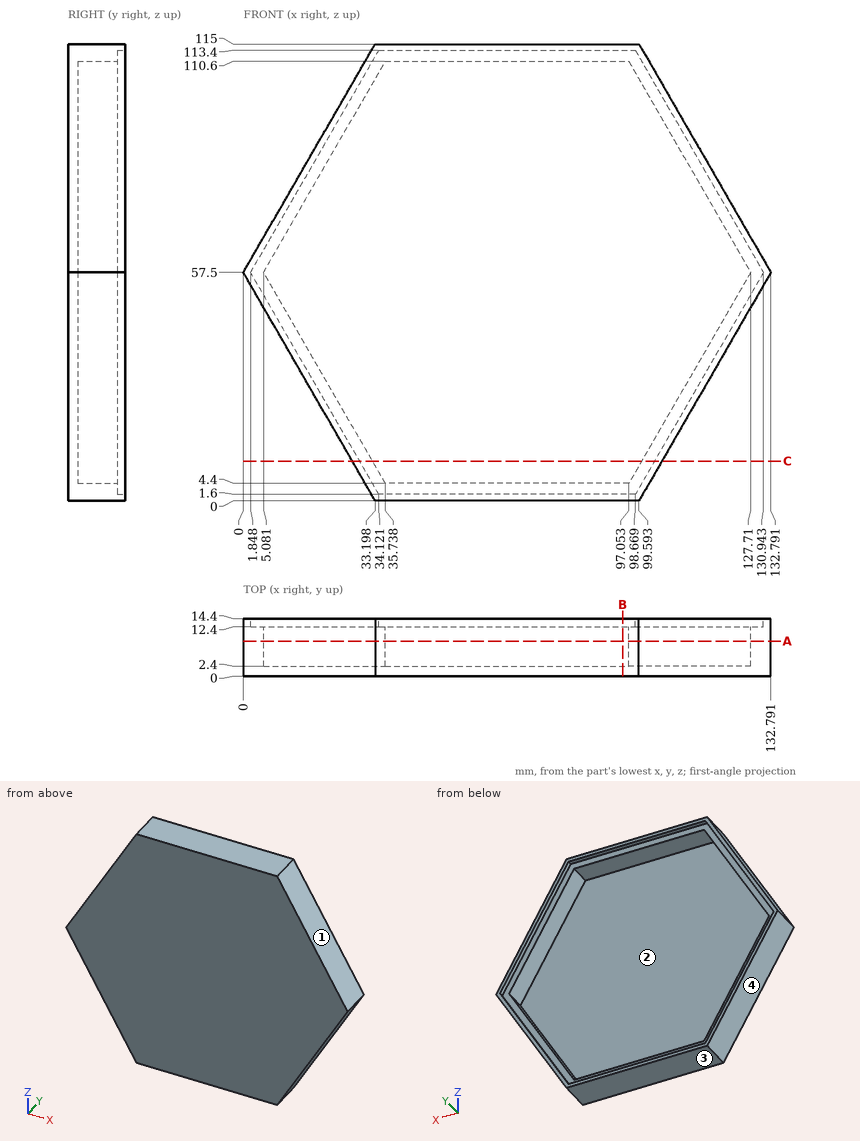
The drawing under review shows one solid part. Ordinate dimensions are in mm from its lowest x, y, z. Round coordinates to 2 decimals unless told otherwise and drop trailing zeros. Loops run counter-clockwise (first coordinate to the right, second up) from the corner with the lowest first, then second, coordinate; pieces in that order, holes last. Notation, with made-up numbers: (81, 80.5) - (102, 80.5) arc R15 ccw to (102, 108.5) - close; hole circle Ø10 at (34.5, 70.5). An arc over 180 degrees is marked (long way). Put each result on its own line as item: value. Start each with the question number.
1. Mouldability with a two-part tool opening along X and no side actions: class the marked faces 1, 2, 3 and 4 as +X half, -X half, draft (parallel to the pull), parting line (faces both ways), or undercut.
2. Insertion check: P1, Ø8, axis at y = 11, z = 81.5, coming from the -X side; P2, Ø6, axis at x = 18, y = 5.5, coming from the -Z side (1 decimal); P3, Ø4, axis at x = 102.5, y = 5.5, coming from the -Z side. Each pin has a flat end and moves straight along its axis. Give the tip position at first contact, or say it passes through.
3. For probe 1 along Z at (x, y) = (93, 9.75); probe 2 along Y at (x, z) = (63, 55.5); probe 3 along X at (y, z) = (9, 80), list the stretches that pass through material, from the lowest coordinate up. Write a range as [from, to].
4. Consider section C-C on z = 10. State the section outline as (x, y) points (1 decimal), plus the area to 3 significant figures.
5. Consider section B-B on x = 95.5. State the section outline as (y, z) points.
6. Consider section A-A on y = 8.75. State the section outline as (x, z) points, plus the area to 3 significant figures.
Result sheet:
1. face 1: +X half
1. face 2: undercut
1. face 3: draft
1. face 4: -X half
2. P1: x = 11.55
2. P2: z = 21.1
2. P3: z = 1.57
3. probe 1: [0, 4.4], [110.6, 115]
3. probe 2: [0, 2.4]
3. probe 3: [12.99, 18.07], [114.72, 119.8]
4. outline: (27.4, 0) - (105.4, 0) - (105.4, 14.4) - (103.5, 14.4) - (103.5, 12.4) - (100.3, 12.4) - (100.3, 2.4) - (32.5, 2.4) - (32.5, 12.4) - (29.3, 12.4) - (29.3, 14.4) - (27.4, 14.4) - close
4. area: 296 mm^2
5. outline: (0, 0) - (14.4, 0) - (14.4, 1.6) - (12.4, 1.6) - (12.4, 4.4) - (2.4, 4.4) - (2.4, 110.6) - (12.4, 110.6) - (12.4, 113.4) - (14.4, 113.4) - (14.4, 115) - (0, 115) - close
6. outline: (0, 57.5) - (33.2, 0) - (99.59, 0) - (132.79, 57.5) - (99.59, 115) - (33.2, 115) - close; hole (5.08, 57.5) - (35.74, 4.4) - (97.05, 4.4) - (127.71, 57.5) - (97.05, 110.6) - (35.74, 110.6) - close
6. area: 1,690 mm^2
